Design review of the part built by this model. Coordinates are the model's own, in mm. Face numbers are marked on the shaded views. A direction names the side the tool comes from. Round coordinates to 2 decimals unless told otherwise and drop trailing zeros. Order: outer loops, then holes, each group sorted by start corner. A loop starts at its lowest first (then second) coordinate and runs counter-clockwise, first axis right, second up. Notation, with made-up numbers: (-7, 37) - (30, 37) arc R10 cw to (30, 46) - close; hole circle Ø1 at (8.5, 88). An arc over 180 degrees is marked (long way). Use CSV: the item, a comma, the result in double quotes.
from build123d import *

# Parameters (mm, degrees)
F0_R         = 7.9375
F1_DEPTH     = 1.5875
F2_R         = 6.35
F3_DEPTH     = 8
F4_W         = 15.875
F4_H         = 15.875
F5_DEPTH     = 6.35
F6_R         = 2.5
F7_DEPTH     = 15.9375
F8_R         = 1.5875
F9_REACH     = 20.3661280605
F10_T1_DEPTH = 46.0375


# Not quite as in the source:
# - a fillet or chamfer that OpenCascade refuses, or shapes differently, is made with other operations: its cross-section is extruded or revolved along the edge and cut away or added


with BuildPart() as f1:
    # F0 (on Top) → F1 (new body)
    with BuildSketch(Plane.XY):
        Circle(F0_R)
    extrude(amount=F1_DEPTH)

    # F2 (on face) → F3 (join)
    with BuildSketch(Plane.XY.offset(1.5875)):
        Circle(F2_R)
    extrude(amount=F3_DEPTH)

    # F4 (on face) → F5 (join)
    with BuildSketch(Plane.XY.offset(9.5875)):
        Rectangle(F4_W, F4_H)
    extrude(amount=F5_DEPTH)

    # F6 (on face) → F7 (cut, through all)
    with BuildSketch(Plane.XY.offset(15.9375)):
        Circle(F6_R)
    extrude(amount=-F7_DEPTH, mode=Mode.SUBTRACT)

    f9_end = f1.faces().sort_by_distance((-2.5, 0, 7.96875))[0]
    # F8 (on face) → F9 (cut, up to a face of the model that its end follows)
    with BuildSketch(Plane(origin=(0, 7.9375, 0), x_dir=(-1, 0, 0), z_dir=(0, 1, 0))):
        with Locations((0, 12.7625)):
            Circle(F8_R)
    f9_long = extrude(amount=-F9_REACH, mode=Mode.PRIVATE)
    add(split(f9_long, bisect_by=f9_end, keep=Keep.ALL, mode=Mode.PRIVATE).solids().sort_by_distance((0, 7.9375, 12.7625))[0], mode=Mode.SUBTRACT)

    # F10: fillet of radius 7.9375 on 4 edges, made by hand

    # F10_s2 → F10_t1 (cut)
    with BuildSketch(Plane.XY.offset(-10.25625)):
        with BuildLine():
            ThreePointArc((-7.9375, 0), (-5.6126600757, 5.6126600757), (0, 7.9375))
            Line((0, 7.9375), (-7.9375, 7.9375))
            Line((-7.9375, 7.9375), (-7.9375, 0))
        make_face()
        with BuildLine():
            ThreePointArc((0, -7.9375), (-5.6126600757, -5.6126600757), (-7.9375, 0))
            Line((-7.9375, 0), (-7.9375, -7.9375))
            Line((-7.9375, -7.9375), (0, -7.9375))
        make_face()
        with BuildLine():
            ThreePointArc((7.9375, 0), (5.6126600757, 5.6126600757), (0, 7.9375))
            Line((0, 7.9375), (7.9375, 7.9375))
            Line((7.9375, 7.9375), (7.9375, 0))
        make_face()
        with BuildLine():
            ThreePointArc((0, -7.9375), (5.6126600757, -5.6126600757), (7.9375, 0))
            Line((7.9375, 0), (7.9375, -7.9375))
            Line((7.9375, -7.9375), (0, -7.9375))
        make_face()
    extrude(amount=F10_T1_DEPTH, mode=Mode.SUBTRACT)


solid = f1.part
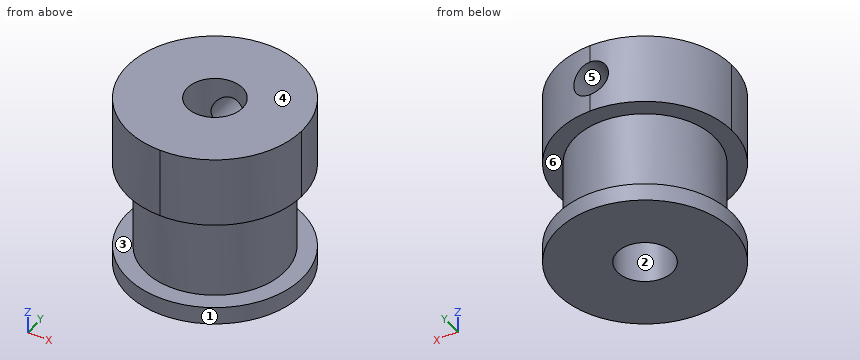
1) For the marked faces 4, 5 and 6, list the 3-axis set-ups (+Z, -Z, +X, -X, +Y, -Y) from which the entire face can be reached by the end or side of a thin tool; tool diameter is ignored.
Data:
face 4,"+Z, +X, -X, +Y, -Y"
face 5,"+Y"
face 6,"none"
2) We need section C-C (x = 1). Give the boundary of the cut face in (y, z), then the cut area to 3 significant figures.
Data:
outline,"(-7.87, 0) - (-2.29, 0) - (-2.29, 15.94) - (-7.87, 15.94) - (-7.87, 9.59) - (-6.27, 9.59) - (-6.27, 1.59) - (-7.87, 1.59) - close; (2.29, 0) - (7.87, 0) - (7.87, 1.59) - (6.27, 1.59) - (6.27, 9.59) - (7.87, 9.59) - (7.87, 11.53) - (2.29, 11.53) - close; (2.29, 14) - (7.87, 14) - (7.87, 15.94) - (2.29, 15.94) - close"
area,"139 mm2"
3) Insertion check: pin 1 Ø4 at (y, z) = (-4.5, 2) entering from +X; pin 2 Ø2 at (x, z) = (5.5, 3.5) entering from +Y; pin 3 Ø2 at (y, z) = (-3.5, 8) entering from -X; pin 4 Ø8 at (x, y) = (0, 0) entering from +Z. Each pin has a flat end and moves straight along its axis. Give the tip position at first contact, or say it passes through.
Data:
pin 1,"stops at x = 7.52"
pin 2,"stops at y = 4.48"
pin 3,"stops at x = -5.84"
pin 4,"stops at z = 15.94"
4) We need section B-B (y = 3.5). Give the boundary of the cut face in (x, z) (1 decimal).
Data:
outline,"(-7.1, 0) - (7.1, 0) - (7.1, 1.6) - (5.3, 1.6) - (5.3, 9.6) - (7.1, 9.6) - (7.1, 15.9) - (-7.1, 15.9) - (-7.1, 9.6) - (-5.3, 9.6) - (-5.3, 1.6) - (-7.1, 1.6) - close; hole circle Ø3.2 at (0, 12.8)"
5) To check wall thickness, follow L1, parallel to Y at x = 0, z = 10.25; L2, parallel to Z at x = -7, y = 0.25; L3, parallel to X at y = 2, z = 12. State the ranges of each line that lie inside material, in increasing order. Write a range as from..to.
Data:
L1,"y = -7.94..-2.5, 2.5..7.94"
L2,"z = 0..1.59, 9.59..15.94"
L3,"x = -7.68..-1.5, 1.5..7.68"
6) The part is to be moulded in two halves that separate along Y. For the marked faces 1, 2 and 3, say which applies: +Y half, -Y half, draft (parallel to the pull), parting line (faces both ways), or undercut.
Data:
face 1,"parting line"
face 2,"undercut"
face 3,"draft"
7) We need section D-D (x = -5). Give the boundary of the cut face in (y, z).
Data:
outline,"(-6.16, 0) - (6.16, 0) - (6.16, 1.59) - (3.91, 1.59) - (3.91, 9.59) - (6.16, 9.59) - (6.16, 15.94) - (-6.16, 15.94) - (-6.16, 9.59) - (-3.91, 9.59) - (-3.91, 1.59) - (-6.16, 1.59) - close"
8) We need section A-A (y = 1.25). Give the boundary of the cut face in (x, z), then the cut area to 3 significant figures.
Data:
outline,"(-7.84, 0) - (-2.17, 0) - (-2.17, 15.94) - (-7.84, 15.94) - (-7.84, 9.59) - (-6.23, 9.59) - (-6.23, 1.59) - (-7.84, 1.59) - close; (2.17, 0) - (7.84, 0) - (7.84, 1.59) - (6.23, 1.59) - (6.23, 9.59) - (7.84, 9.59) - (7.84, 15.94) - (2.17, 15.94) - close"
area,"155 mm2"
